```python
from build123d import *

# Parameters (mm, degrees)
SKETCH1_R                        = 6.35
SKETCH1_R_2                      = 3.96875
BOSS_EXTRUDE1_DEPTH              = 3.175
SKETCH2_R                        = 6.35
CUT_EXTRUDE1_DEPTH               = 0.254
F_1_4_20_TAPPED_HOLE1_AT_2_COUNT = 2
F_1_4_20_TAPPED_HOLE1_AT_2_PITCH = 43.994090512
F_1_4_20_TAPPED_HOLE1_AT_3_COUNT = 2
F_1_4_20_TAPPED_HOLE1_AT_3_PITCH = 43.994090512


with BuildPart() as part:
    # Sketch1 → Boss-Extrude1 (new body)
    with BuildSketch(Plane(origin=(0, 0, 0), x_dir=(1, 0, 0), z_dir=(0, 1, 0))):
        Polygon((0, 0), (139.954, 0), (69.977, 121.203719361), align=None)
        with Locations((69.977, 40.401239787)):
            Circle(SKETCH1_R, mode=Mode.SUBTRACT)
        with Locations((117.956954744, 12.7)):
            Circle(SKETCH1_R_2, mode=Mode.SUBTRACT)
        with Locations((21.997045256, 12.7)):
            Circle(SKETCH1_R_2, mode=Mode.SUBTRACT)
        with Locations((69.977, 95.803719361)):
            Circle(SKETCH1_R_2, mode=Mode.SUBTRACT)
    extrude(amount=BOSS_EXTRUDE1_DEPTH)

    # Sketch2 → Cut-Extrude1 (cut)
    with BuildSketch(Plane(origin=(0, 0, 0), x_dir=(1, 0, 0), z_dir=(0, 1, 0))):
        with Locations((93.966977372, 54.251859681)):
            Circle(SKETCH2_R)
        with Locations((69.977, 12.7)):
            Circle(SKETCH2_R)
        with Locations((45.987022628, 54.251859681)):
            Circle(SKETCH2_R)
    extrude(amount=CUT_EXTRUDE1_DEPTH, mode=Mode.SUBTRACT)

    # Sketch4 → 1/4-20 Tapped Hole1 (revolve, cut)
    with BuildSketch(Plane(origin=(56.837296951, 3.175, -18.663985964), x_dir=(0, 0, 1), z_dir=(1, 0, 0))):
        Polygon((0, 0), (0, 3.175), (2.5527, 3.175), (2.5527, 1.054999966), (3.81, 0), align=None)
    f_1_4_20_tapped_hole1 = revolve(axis=Axis((56.837296951, 9.525, -18.663985964), (0, -1, 0)), mode=Mode.SUBTRACT)

    # 1/4-20 Tapped Hole1 at 2: 1/4-20 Tapped Hole1 ×2
    with Locations(*[Vector(0.875903289, 0, -0.482486712) * (i * F_1_4_20_TAPPED_HOLE1_AT_2_PITCH) for i in range(1, F_1_4_20_TAPPED_HOLE1_AT_2_COUNT)]):
        add(f_1_4_20_tapped_hole1, mode=Mode.SUBTRACT)

    # 1/4-20 Tapped Hole1 at 3: 1/4-20 Tapped Hole1 ×2
    with Locations(*[Vector(0.020105895, 0, -0.999797856) * (i * F_1_4_20_TAPPED_HOLE1_AT_3_PITCH) for i in range(1, F_1_4_20_TAPPED_HOLE1_AT_3_COUNT)]):
        add(f_1_4_20_tapped_hole1, mode=Mode.SUBTRACT)


solid = part.part
```
Part model, mm, in its own coordinate system. A direction names the side the tool comes from. Round coordinates to 2 decimals unless told otherwise and drop trailing zeros. Order: outer loops, then holes, each group sorted by start corner. A loop starts at its lowest first (then second) coordinate and runs counter-clockwise, first axis right, second up. Notation, with made-up numbers: M 75,26.5 L 128,26.5 A23 cw 128,38.5 Z; hole C 81,25 d7. An arc over 180 degrees is marked long. Put each result on its own line as item: value. Start each with the question number.
1. Slice it at D-D on z = -109.5. List the corners of the cut face in (x, y) (3 decimals).
2. Two-plate mould, pull along X, no slides. Class faces 1 (the face through (105.455, 1.565, -59.753)), 2 (the face through (18.03, 1.57, -12.87)), 3 (the face through (94, 0.254, -54)), 4 (the face through (69, 3.175, -48)): +X half, -X half, draft (parallel to the pull), parting line (faces both ways), or undercut.
3. Drop flat-ended pins along their axis: pin 1 (10 mm diameter, centred on x = 70.5, z = -11.5, fed in from -Y); pin 2 (1.5 mm diameter, centred on y = 0.5, z = -100.5, fed in from -X); pin 3 (10 mm diameter, centred on x = 92.5, z = -54, fed in from -Y); pin 4 (4.5 mm diameter, centred on x = 57.72, z = -62.65, fed in from +Y). Give the stop position or say it passes through.
4. Slice it at C-C on x = 119. List the corners of the cut face in (y, z) (3 decimals), then the cut area to 3 significant figures.
5. Tool access for faces 5 (the face through (73.64, 1.57, -94.28)), 6 (the face through (46, 0.254, -54)): list every direction of +Z, -Z, +X, -X, +Y, -Y with a clear straight run to the whole face (end or side of a thin tool).
6. Slice it at A-A on y = 1.25. List the corners of the cut face in (x, z).
7. Slice it at B-B on z = -12.7. List the corners of the cut face in (x, y) (3 decimals).
8. Drill centre lines: probe 1 along X at (y, z) = (1.15, -38); probe 2 along X at (y, z) = (0.95, -12.7); probe 3 along Z at (x, y) = (55.5, 1.8). Where is each one in solid material? Low to high. Write a range as [from, to].
Findings:
1. outline: M 63.22,0 L 76.734,0 L 76.734,3.175 L 63.22,3.175 Z
2. face 1: +X half
2. face 2: undercut
2. face 3: undercut
2. face 4: draft
3. pin 1: y = 0.25
3. pin 2: x = 57.59
3. pin 3: y = 0
3. pin 4: through
4. outline: M 0,-36.293 L 3.175,-36.293 L 3.175,-16.529 L 0,-16.529 Z; M 0,-8.871 L 3.175,-8.871 L 3.175,0 L 0,0 Z
4. area: 90.9 mm2
5. face 5: +Y, -Y
5. face 6: -Y
6. outline: M 0,0 L 69.98,-121.2 L 139.95,0 Z; hole C 22,-12.7 d7.94; hole C 56.84,-18.66 d5.11; hole C 57.72,-62.65 d5.11; hole C 69.98,-40.4 d12.7; hole C 69.98,-95.8 d7.94; hole C 95.37,-39.89 d5.11; hole C 117.96,-12.7 d7.94
7. outline: M 7.332,0 L 18.028,0 L 18.028,3.175 L 7.332,3.175 Z; M 25.966,0 L 63.627,0 L 63.627,0.254 L 76.327,0.254 L 76.327,0 L 113.988,0 L 113.988,3.175 L 25.966,3.175 Z; M 121.926,0 L 132.622,0 L 132.622,3.175 L 121.926,3.175 Z
8. probe 1: [21.94, 64.1], [75.86, 93.66], [97.09, 118.01]
8. probe 2: [7.33, 18.03], [25.97, 113.99], [121.93, 132.62]
8. probe 3: [-96.13, -63.91], [-61.39, -20.84], [-16.49, 0]
